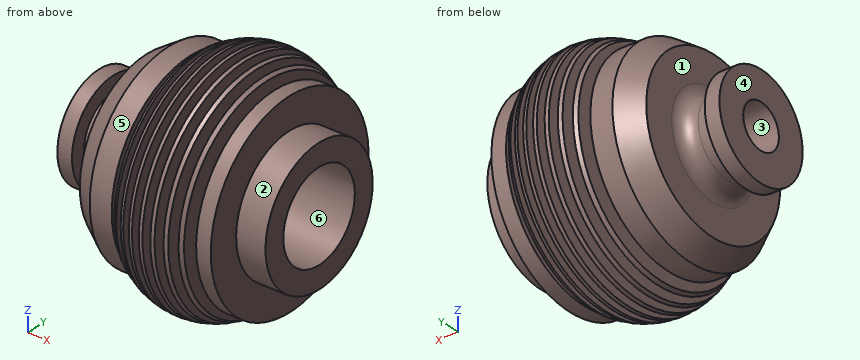
from build123d import *


with BuildPart() as part:
    # Sketch1 → Revolve1 (revolve)
    with BuildSketch(Plane.XY, mode=Mode.PRIVATE) as revolve1_sk:
        with BuildLine():
            ThreePointArc((25, 59.33620738), (26.242582391, 59.827647663), (27.5, 60.279782054))
            Line((27.5, 60.279782054), (27.5, 35.065472262))
            Line((27.5, 35.065472262), (32.5, 35.065472262))
            Line((32.5, 35.065472262), (32.5, 61.655024098))
            ThreePointArc((32.5, 61.655024098), (33.746649446, 61.897912685), (35, 62.103441501))
            Line((35, 62.103441501), (35, 35.065472262))
            Line((35, 35.065472262), (40, 35.065472262))
            Line((40, 35.065472262), (40, 62.547125869))
            ThreePointArc((40, 62.547125869), (41.25, 62.565512199), (42.5, 62.547125869))
            Line((42.5, 62.547125869), (42.5, 35.065472262))
            Line((42.5, 35.065472262), (47.5, 35.065472262))
            Line((47.5, 35.065472262), (47.5, 62.103441501))
            ThreePointArc((47.5, 62.103441501), (48.753350554, 61.897912685), (50, 61.655024098))
            Line((50, 61.655024098), (50, 35.065472262))
            Line((50, 35.065472262), (55, 35.065472262))
            Line((55, 35.065472262), (55, 60.279782054))
            ThreePointArc((55, 60.279782054), (56.257417609, 59.827647663), (57.5, 59.33620738))
            Line((57.5, 59.33620738), (57.5, 35.065472262))
            Line((57.5, 35.065472262), (62.5, 35.065472262))
            Line((62.5, 35.065472262), (62.5, 56.871591859))
            ThreePointArc((62.5, 56.871591859), (63.76354019, 56.112571831), (65, 55.310192648))
            Line((65, 55.310192648), (65, 35.065472262))
            Line((65, 35.065472262), (70, 35.065472262))
            Line((70, 35.065472262), (70, 51.365472262))
            Line((70, 51.365472262), (80, 51.365472262))
            Line((80, 51.365472262), (80, 30.065472262))
            Line((80, 30.065472262), (100, 30.065472262))
            Line((100, 30.065472262), (100, 15.065472262))
            Line((100, 15.065472262), (0, 15.065472262))
            Line((0, 15.065472262), (0, 0))
            Line((0, 0), (-21.679197995, 0))
            Line((-21.679197995, 0), (-50, 0))
            Line((-50, 0), (-50, 20))
            Line((-50, 20), (-40, 20))
            Line((-40, 20), (-40, 10))
            Line((-40, 10), (-27.422676306, 10))
            ThreePointArc((-27.422676306, 10), (-20.351608494, 12.928932188), (-17.422676306, 20))
            Line((-17.422676306, 20), (-17.422676306, 41.3))
            Line((-17.422676306, 41.3), (-2.5, 51.365472262))
            Line((-2.5, 51.365472262), (12.5, 51.365472262))
            Line((12.5, 51.365472262), (12.5, 35.065472262))
            Line((12.5, 35.065472262), (17.5, 35.065472262))
            Line((17.5, 35.065472262), (17.5, 55.310192648))
            ThreePointArc((17.5, 55.310192648), (18.73645981, 56.112571831), (20, 56.871591859))
            Line((20, 56.871591859), (20, 35.065472262))
            Line((20, 35.065472262), (25, 35.065472262))
            Line((25, 35.065472262), (25, 59.33620738))
        make_face()
    revolve(revolve1_sk.sketch.rotate(Axis((-50, -15, 0), (1, 0, 0)), 90), axis=Axis((-50, -15, 0), (1, 0, 0)))


solid = part.part
Check sheet for the modelled part. Datum: model origin and axes. Units: mm. Face numbers are marked on the shaded views. A direction names the side the tool comes from. Round coordinates to 2 decimals unless told otherwise and drop trailing zeros. Loops run counter-clockwise (first coordinate to the right, second up) from the corner with the lowest first, then second, coordinate; pieces in that order, holes last. Notation, with made-up numbers: (28.5, -29) -> (52.5, -29) arc R7 cw to (52.5, -23) -> close; hole circle Ø7 at (85.5, -34). An arc over 180 degrees is marked (long way). Put each result on its own line as item: value. Start each with the question number.
1. Draft check along Z on the marked faces 1, 2 and 3. Enter one of: +Z half, -Z half, draft (parallel to the pull), parting line (faces both ways), or undercut.
2. Section check C-C (x = 7.5). Enter the section's corners in (y, z), plus the area to 3 significant figures.
3. Access from +Z, -Z, +X, -X, +Y, -Y to the whole of each face (thin tool, end or side, straight path). Record for the marked faces 4, 5 and 6.
4. Scan lines: probe 1 along X at (y, z) = (-74.5, -40.5); probe 2 along Y at (x, z) = (44, 0); probe 3 along Y at (x, z) = (-28, 0). Record each from-to range of solid material in increasing order.
5. Section check B-B (z = -59). Give the number of separate pieces and of enclosed holes in the cut face, plus the area to 3 significant figures.
6. Gauge pin test, flat ends, axial feed: pin 1 (4 mm diameter, centred on y = -1.5, z = -7.5, fed in from +X); pin 2 (12 mm diameter, centred on x = 50.5, y = 5.5, fed in from +Z); pin 3 (10 mm diameter, centred on y = 40.5, z = -61, fed in from +X). Record the tip position at first contact, or that the pin passes through.
7. Section check A-A (x = -32.5). Enter the section's corners in (y, z).
Findings:
1. face 1: draft
1. face 2: parting line
1. face 3: undercut
2. outline: circle Ø132.73 at (-15, 0); hole circle Ø60.13 at (-15, 0)
2. area: 11,000 mm^2
3. face 4: +Z, -Z, -X, +Y, -Y
3. face 5: -X
3. face 6: +X
4. probe 1: x = 25 to 27.5, 32.5 to 35, 40 to 42.5, 47.5 to 50, 55 to 57.5
4. probe 2: y = -65.07 to -45.07, 15.07 to 35.07
4. probe 3: y = -40 to -30, 0 to 10
5. separate pieces: 9
5. enclosed holes: 0
5. area: 3,560 mm^2
6. pin 1: stops at x = 0
6. pin 2: stops at z = 75.57
6. pin 3: stops at x = 42.5
7. outline: circle Ø50 at (-15, 0); hole circle Ø30 at (-15, 0)
